Check sheet for the drawn part. Datum: minimum x, y, z corner. Units: mm. A direction names the side the tool comes from. Give positions to 0.01 mm unless a question says otherwise; leave off trailing zeros. Loops run counter-clockwise (first coordinate to the right, second up) from the corner with the lowest first, then second, coordinate; pieces in that order, holes last.
1. Cross-section at A-A, the plane y = 20. Record the cut outline in (x, z), plus the area to 3 significant figures.
2. Tool access check on the marked faces 1, 2, 3 and 4. Record the directions out of +Z, -Z, +X, -X, +Y, -Y that give a thin tool (end or side, any length) a straight path to the whole face; none if there is none.
3. Release check for a two-part mould opening along Z. For the marked faces 5, 6, 7 and 8 record: +Z half, -Z half, draft (parallel to the pull), parting line (faces both ways), or undercut.
4. Cross-section at C-C, the plane y = 34. Record the cut outline in (x, z).
5. Go/stop test with flat-tipped pins: pin 1 Ø3 at (x, z) = (20.5, 21) entering from -Y; pin 2 Ø10 at (y, z) = (7, 18.5) entering from -X; pin 3 Ø9 at (x, y) = (20, 20) entering from +Z; pin 4 Ø3 at (y, z) = (18.5, 21.5) entering from -X. Record where each tip stops, or that it passes through.
6. Material ranges on L1, parallel to Z at x = 36.25, y = 20; L2, parallel to X at y = 18, z = 5.5, recorded low to high.
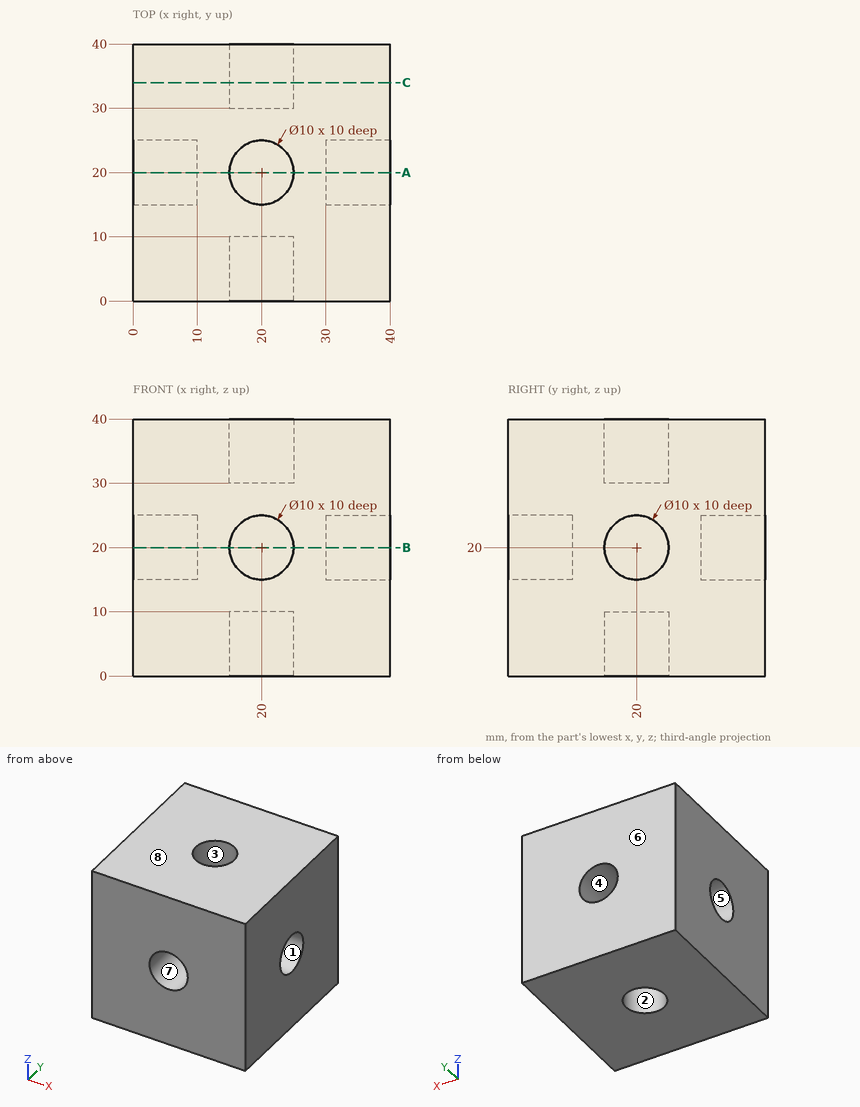
Result:
1. outline: (0, 0) - (15, 0) - (15, 10) - (25, 10) - (25, 0) - (40, 0) - (40, 15) - (30, 15) - (30, 25) - (40, 25) - (40, 40) - (25, 40) - (25, 30) - (15, 30) - (15, 40) - (0, 40) - (0, 25) - (10, 25) - (10, 15) - (0, 15) - close
1. area: 1,200 mm2
2. face 1: +X
2. face 2: -Z
2. face 3: +Z
2. face 4: +Y
3. face 5: undercut
3. face 6: draft
3. face 7: undercut
3. face 8: +Z half
4. outline: (0, 0) - (40, 0) - (40, 40) - (0, 40) - close; hole circle Ø10 at (20, 20)
5. pin 1: stops at y = 10
5. pin 2: stops at x = 0
5. pin 3: stops at z = 30
5. pin 4: stops at x = 10
6. L1: z = 0 to 15, 25 to 40
6. L2: x = 0 to 15.42, 24.58 to 40
